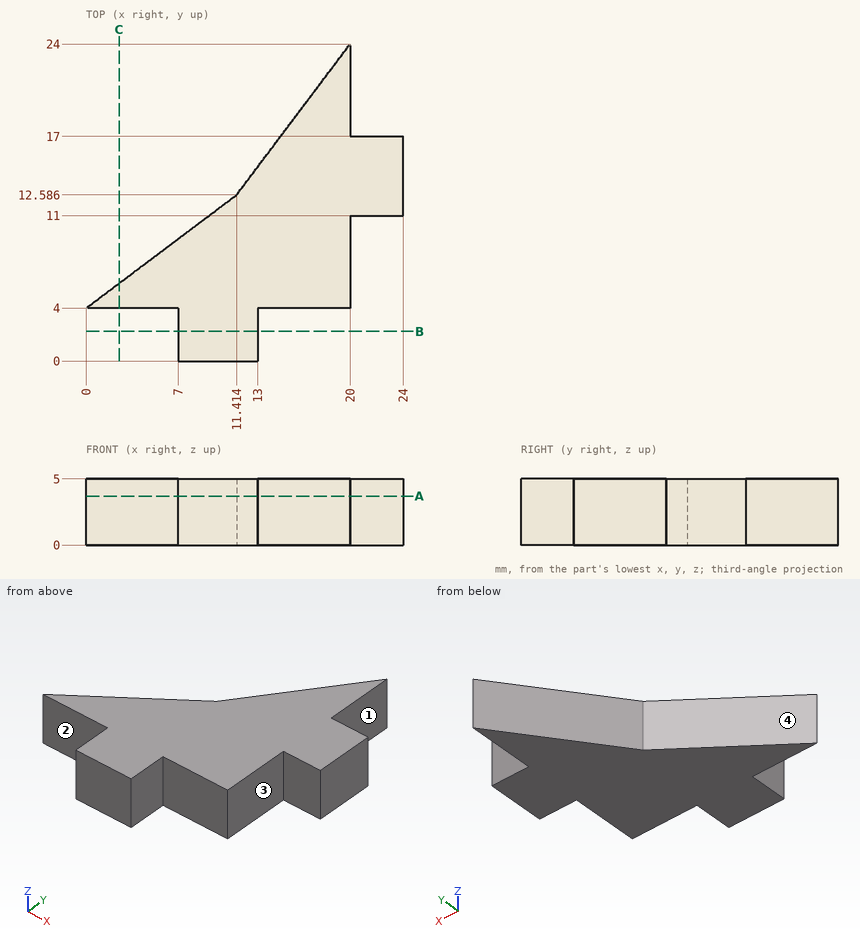
Job drawing, mm, ordinate dimensions from the low corner. One solid piece. A direction names the side the tool comes from. Give positions to 0.01 mm unless a question says otherwise; leave off trailing zeros. Write each loop counter-clockwise with the first axis right and the second up, starting at its lowest first coordinate (ties: lowest second). Pieces come first, ordered by that corner, then holes. Notation, with made-up numbers: (19, 73.5) - (77, 73.5) arc R21 ccw to (77, 106.5) - close; hole circle Ø1 at (87.25, 79). An arc over 180 degrees is marked (long way). Use one line per item in the form item = value. Start each with the question number.
1. Band-saw the part on B-B on y = 2.25. Write the cut outline in (x, z).
2. Band-saw the part on C-C on x = 2.5. Write the cut outline in (y, z).
3. Probe line 1 (Y direction, x = 20.5, z = 1.1); line 2 (X direction, y = 3.75, z = 3.85); line 3 (Y direction, x = 4.75, z = 3.85). List the from-to ranges inside material, lowest first. Write a range as [from, to].
4. 3-axis set-ups, long thin cutter, end or side, ignore diameter. For the marked faces 1, 2, 3 and 4: which of +Z, -Z, +X, -X, +Y, -Y reach the whole face in a straight line?
5. Drop flat-ended pins along their axis: pin 1 Ø1.5 at (y, z) = (20, 2) entering from -X; pin 2 Ø1.5 at (y, z) = (10.5, 3) entering from +X; pin 3 Ø2 at (y, z) = (4, 4.5) entering from +X; pin 4 Ø1.2 at (x, z) = (22.5, 3) entering from +Y. Give the stop position or say it passes through.
6. Band-saw the part on A-A on z = 3.7. Write the cut outline in (x, y), plus the area to 3 significant figures.
Conclusion:
q1.outline = (7, 0) - (13, 0) - (13, 5) - (7, 5) - close
q2.outline = (4, 0) - (5.88, 0) - (5.88, 5) - (4, 5) - close
q3.line_1 = [11, 17]
q3.line_2 = [7, 13]
q3.line_3 = [4, 7.57]
q4.face_1 = +Z, -Z, +X, +Y
q4.face_2 = +Z, -Z, -X, -Y
q4.face_3 = +Z, -Z, +X, -Y
q4.face_4 = +Z, -Z, -X, +Y
q5.pin_1 = 16.43
q5.pin_2 = 24
q5.pin_3 = 20
q5.pin_4 = 17
q6.outline = (0, 4) - (7, 4) - (7, 0) - (13, 0) - (13, 4) - (20, 4) - (20, 11) - (24, 11) - (24, 17) - (20, 17) - (20, 24) - (11.41, 12.59) - close
q6.area = 220 mm²
